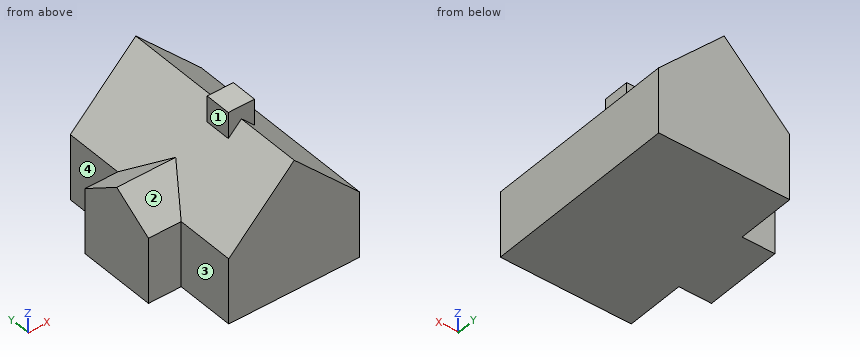
```python
from build123d import *

# Parameters (mm, degrees)
F1_DEPTH      = 150
F3_DEPTH      = 25
F3_DEPTH_BACK = 25
F5_W          = 20
F5_H          = 20
F6_DEPTH      = 20


with BuildPart() as f1:
    # F0 (on Front) → F1 (new body)
    with BuildSketch(Plane.XZ):
        Polygon((0, 50), (0, 0), (100, 0), (100, 50), (50, 100), align=None)
    extrude(amount=F1_DEPTH)

    # F2 (on face) → F3 (join, two sides)
    with BuildSketch(Plane(origin=(0, 0, 0), x_dir=(0, -1, 0), z_dir=(-1, 0, 0))) as f3_sk:
        Polygon((45, 50), (45, 0), (105, 0), (105, 50), (75, 70), align=None)
    extrude(amount=F3_DEPTH)
    extrude(f3_sk.sketch, amount=-F3_DEPTH_BACK)

    # F5 (on offset) → F6 (join)
    with BuildSketch(Plane.XZ.offset(100)):
        with Locations((50, 100)):
            Rectangle(F5_W, F5_H)
    extrude(amount=-F6_DEPTH)


solid = f1.part
```
Read the model definition and answer for the solid it produces. Units are mm, in the model's axes. Face numbers are marked on the shaded views. A direction names the side the tool comes from. Give positions to 0.01 mm unless a question says otherwise; leave off trailing zeros. Order: outer loops, then holes, each group sorted by start corner. A loop starts at its lowest first (then second) coordinate and runs counter-clockwise, first axis right, second up.
(1) Find section A-A (x = 7.5). Give the vertices of the cut face in (y, z).
(2) For the marked faces 1, 2, 3 and 4, determine the directions among +Z, -Z, +X, -X, +Y, -Y from which every point of the face is accessible in a straight line to the end or side of a thin tool.
(3) Find section C-C (z = 24.5). Give the vertices of the cut face in (x, y).
(4) Find section B-B (y = -115). Give the vertices of the cut face in (x, z).
(5) Given pin 1 (22.5 mm diameter, centred on y = -123.5, z = 31.5, fed in from -X); pin 2 (1.5 mm diameter, centred on y = -102, z = 71, fed in from -X); pin 3 (6 mm diameter, centred on x = 39.5, y = -54.5, fed in from +Z), each flat-ended and moving along its own axis, determine where each tip first touches the part or whether it passes through.
(6) Straight lines are drawn through the part: L1, parallel to Y at x = 43, z = 97; L2, parallel to X at y = -140.5, z = 11; L3, parallel to X at y = -19, z = 90. For each, find the intervals that lie inside material, in ascending order.
(7) Find section D-D (x = 83.5). Give the vertices of the cut face in (y, z), plus the area to 4 significant figures.
Result sheet:
1. outline: (-150, 0) - (0, 0) - (0, 57.5) - (-56.25, 57.5) - (-75, 70) - (-93.75, 57.5) - (-150, 57.5) - close
2. face 1: +Z, -X, +Y, -Y
2. face 2: +Z, -X, -Y
2. face 3: +Z, -Z, -X, -Y
2. face 4: +Z, -Z, -X, +Y
3. outline: (-25, -105) - (0, -105) - (0, -150) - (100, -150) - (100, 0) - (0, 0) - (0, -45) - (-25, -45) - close
4. outline: (0, 0) - (100, 0) - (100, 50) - (50, 100) - (0, 50) - close
5. pin 1: stops at x = 0
5. pin 2: stops at x = 20.25
5. pin 3: stops at z = 92.5
6. L1: y = -100 to -80
6. L2: x = 0 to 100
6. L3: x = 40 to 60
7. outline: (-150, 0) - (0, 0) - (0, 66.5) - (-150, 66.5) - close
7. area: 9,975 mm2
